The drawing under review shows one solid part. Ordinate dimensions are in mm from its lowest x, y, z. A direction names the side the tool comes from. Round coordinates to 2 decimals unless told otherwise and drop trailing zeros. Order: outer loops, then holes, each group sorted by start corner. A loop starts at its lowest first (then second) coordinate and runs counter-clockwise, first axis right, second up. Notation, with made-up numbers: (-5.5, 80.5) -> (23.5, 80.5) arc R4 cw to (23.5, 87.5) -> close; hole circle Ø4 at (29, -3.75). An arc over 180 degrees is marked (long way). Use a Markdown table: item, result. Add a question column.
1) Consider section B-B (z = 9.5). State the section outline as (x, y) points, plus the area to 3 significant figures.
2) Consider section A-A (y = 28). State the section outline as (x, z) points, plus the area to 3 significant figures.
3) Wall thickness on line 1 along Y through (x, z) = (6, 38.5); line 2 along Y through (x, z) = (19.2, 17); line 3 along Z through (x, y) = (19.2, 38): over which ranges is each line inside the solid? List them lowest first. Write a range as [from, to].
4) Clearance check with flat-ended pins moving along their axes: P1, Ø1.5, axis at x = 11.5, y = 12.5, coming from the -Z side; P2, Ø2, axis at y = 38, z = 17, coming from the +X side. State where each tip first meets the part, or that it passes through.
5) Consider section C-C (x = 6). State the section outline as (y, z) points, plus the area to 3 significant figures.
6) Consider section D-D (y = 40.5). State the section outline as (x, z) points.
7) Machinability: for the marked faces 1 and 2, which of the approach directions +Z, -Z, +X, -X, +Y, -Y give a long, thin tool a straight path to every point of the face, cutting with its end or side? Answer none if there is none.
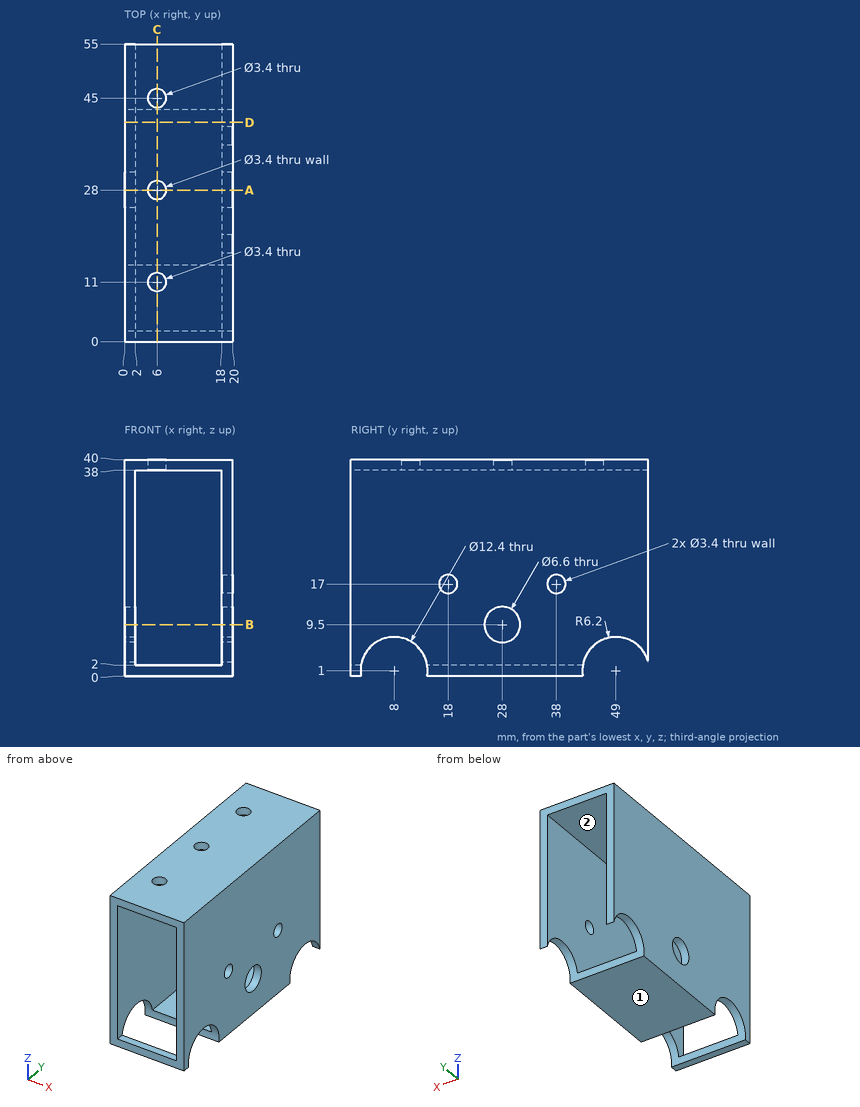
Results list:
| question | item | result |
|---|---|---|
| 1 | outline | (0, 0) -> (2, 0) -> (2, 24.7) -> (0, 24.7) -> close; (0, 31.3) -> (2, 31.3) -> (2, 55) -> (0, 55) -> close; (18, 0) -> (20, 0) -> (20, 24.7) -> (18, 24.7) -> close; (18, 31.3) -> (20, 31.3) -> (20, 55) -> (18, 55) -> close |
| 1 | area | 194 mm2 |
| 2 | outline | (0, 0) -> (20, 0) -> (20, 6.2) -> (18, 6.2) -> (18, 2) -> (2, 2) -> (2, 6.2) -> (0, 6.2) -> close; (0, 12.8) -> (2, 12.8) -> (2, 38) -> (4.3, 38) -> (4.3, 40) -> (0, 40) -> close; (7.7, 38) -> (18, 38) -> (18, 12.8) -> (20, 12.8) -> (20, 40) -> (7.7, 40) -> close |
| 2 | area | 191 mm2 |
| 3 | line 1 | [0, 9.3], [12.7, 26.3], [29.7, 43.3], [46.7, 55] |
| 3 | line 2 | [0, 16.3], [19.7, 36.3], [39.7, 55] |
| 3 | line 3 | [0, 15.3], [18.7, 40] |
| 4 | P1 | z = 38 |
| 4 | P2 | x = 2 |
| 5 | outline | (0, 0) -> (1.88, 0) arc R6.2 cw to (1.88, 2) -> (0, 2) -> close; (0, 38) -> (9.3, 38) -> (9.3, 40) -> (0, 40) -> close; (12.7, 38) -> (26.3, 38) -> (26.3, 40) -> (12.7, 40) -> close; (14.12, 0) -> (42.88, 0) arc R6.2 cw to (42.88, 2) -> (14.12, 2) arc R6.2 cw to start; (29.7, 38) -> (43.3, 38) -> (43.3, 40) -> (29.7, 40) -> close; (46.7, 38) -> (55, 38) -> (55, 40) -> (46.7, 40) -> close |
| 5 | area | 151 mm2 |
| 6 | outline | (0, 0) -> (20, 0) -> (20, 40) -> (0, 40) -> close; hole (2, 2) -> (18, 2) -> (18, 38) -> (2, 38) -> close |
| 7 | face 1 | -Z, +X, -X, +Y, -Y |
| 7 | face 2 | +Y, -Y |
